```python
from build123d import *

# Parameters (mm, degrees)
ESQUISSE1_R        = 17
BOSS_EXTRU_1_DEPTH = 2
ESQUISSE2_R        = 13.78
ESQUISSE2_R_2      = 11
BOSS_EXTRU_2_DEPTH = 5
ESQUISSE3_R        = 15
BOSS_EXTRU_3_DEPTH = 0.25
D_ME1_FACE_RADIUS  = 15
D_ME1_HEIGHT       = 10
D_ME2_FACE_RADIUS  = 11
D_ME2_HEIGHT       = 11
CONG_1_R           = 0.25


with BuildPart() as part:
    # Esquisse1 → Boss.-Extru.1 (new body)
    with BuildSketch(Plane.XY):
        Circle(ESQUISSE1_R)
    extrude(amount=BOSS_EXTRU_1_DEPTH)

    # Esquisse2 → Boss.-Extru.2 (add)
    with BuildSketch(Plane(origin=(0, 0, 0), x_dir=(-1, 0, 0), z_dir=(0, 0, -1))):
        with Locations(Location((0, 0, 0), (0, 0, 180))):
            Circle(ESQUISSE2_R)
        Circle(ESQUISSE2_R_2, mode=Mode.SUBTRACT)
    extrude(amount=BOSS_EXTRU_2_DEPTH)

    # Esquisse3 → Boss.-Extru.3 (add)
    with BuildSketch(Plane.XY.offset(2)):
        Circle(ESQUISSE3_R)
    extrude(amount=BOSS_EXTRU_3_DEPTH)

    # Dôme1: a dome of height H over a round flat face of radius A is a cap of a sphere of radius (A * A + H * H) / (2 * H)
    d_me1_r = (D_ME1_FACE_RADIUS * D_ME1_FACE_RADIUS + D_ME1_HEIGHT * D_ME1_HEIGHT) / (2 * D_ME1_HEIGHT)
    d_me1_base = Plane((0, 0, 2.25), z_dir=(0, 0, 1))
    with Locations(d_me1_base.offset(D_ME1_HEIGHT - d_me1_r)):
        d_me1_ball = Sphere(d_me1_r, mode=Mode.PRIVATE)
    add(split(d_me1_ball, bisect_by=d_me1_base, keep=Keep.TOP, mode=Mode.PRIVATE))

    # Dôme2: a dome of height H over a round flat face of radius A is a cap of a sphere of radius (A * A + H * H) / (2 * H)
    d_me2_r = (D_ME2_FACE_RADIUS * D_ME2_FACE_RADIUS + D_ME2_HEIGHT * D_ME2_HEIGHT) / (2 * D_ME2_HEIGHT)
    d_me2_base = Plane((0, 0, 0), z_dir=(0, 0, 1))
    with Locations(d_me2_base.offset(D_ME2_HEIGHT - d_me2_r)):
        d_me2_ball = Sphere(d_me2_r, mode=Mode.PRIVATE)
    add(split(d_me2_ball, bisect_by=d_me2_base, keep=Keep.TOP, mode=Mode.PRIVATE), mode=Mode.SUBTRACT)

    # Congé1
    cong_1_edges = [part.edges().sort_by_distance(p)[0] for p in [
        (-15, 0, 2),
        (-17, 0, 2),
    ]]
    fillet(cong_1_edges, radius=CONG_1_R - 0.0001)  # a hair under: the kernel refuses the full size


solid = part.part
```
Could you check a few things on this model? Use its own coordinates, in mm. A direction names the side the tool comes from. Coordinates: 2 decimals unless noted, no trailing zeros. Order: outer loops, then holes, each group sorted by start corner. A loop starts at its lowest first (then second) coordinate and runs counter-clockwise, first axis right, second up. Notation, with made-up numbers: M -17.75,-25.75 L -7.75,-25.75 A16 ccw -7.75,-2.75 Z; hole C 43,-28 d11. An arc over 180 degrees is marked long. Use a Markdown table: item, result. Add a question column.
Q1. We'd pull the mould along X, two halves only. Please class faces 1 (the flat face through (-1.1, 11.2, -5)), 2 (the cylindrical face through (2.38, -10.74, -2.46)), 3 (the cylindrical face through (-2.99, 13.45, -2.46)): pulls with the +X half, pulls with the -X half, needs draft (parallel to the pull), parting line crosses it, or undercut.
Q2. I'm going to push flat-ended pins straight in: pin 1 (8 mm diameter, centred on y = 10, z = 9, fed in from -X); pin 2 (4 mm diameter, centred on y = -3.5, z = -2.5, fed in from -X); pin 3 (1.5 mm diameter, centred on x = -9.5, z = 0.5, fed in from +Y). Where does each tip first touch, or does it pass through?
Q3. If I drill on L1, parallel to Y at x = 0, z = -2.6; L2, parallel to Y at x = -0.5, z = 4.75; L3, parallel to X at y = 7, z = -4, over which ranges is the centre line in solid material (lowest first)?
Q4. I want a section at B-B on z = -1.25. List the corners of the cut face in (x, y) for me.
Q5. Which directions (+Z, -Z, +X, -X, +Y, -Y) give clear straight access to the entire face, cutting with the end or side of a thin tool? Please do faces 4 (the flat face through (0, 14, 0)), 5 (the flat face through (4, -15, 2)), 6 (the cylindrical face through (9.139, 14.334, 0.863)).
Q6. I want a section at D-D on z = 5.5. List the corners of the cut face in (x, y) for me.
Checked values:
| question | item | result |
|---|---|---|
| 1 | face 1 | needs draft |
| 1 | face 2 | undercut |
| 1 | face 3 | parting line crosses it |
| 2 | pin 1 | x = -10.5 |
| 2 | pin 2 | x = -13.7 |
| 2 | pin 3 | y = 14.58 |
| 3 | L1 | -13.78 to -11, 11 to 13.78 |
| 3 | L2 | -13.68 to -9.91, 9.91 to 13.68 |
| 3 | L3 | -11.87 to -8.49, 8.49 to 11.87 |
| 4 | outline | C 0,0 d27.56; hole C 0,0 d22 |
| 5 | face 4 | -Z |
| 5 | face 5 | +Z |
| 5 | face 6 | +Z, -Z |
| 6 | outline | C 0,0 d26.37; hole C 0,0 d19.05 |
